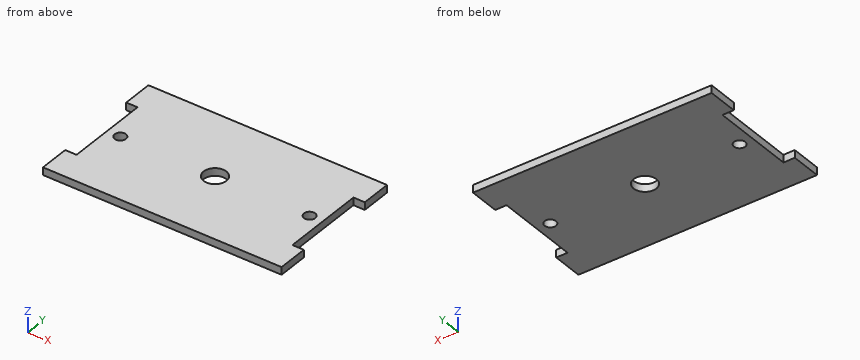
```python
from build123d import *

# Parameters (mm, degrees)
SKETCH_1_R      = 3
SKETCH_1_R_2    = 1.5
EXTRUDE_1_DEPTH = 2


with BuildPart() as part:
    # 草图1 → 凸台-拉伸1 (new body)
    with BuildSketch(Plane.XY):
        Polygon((-13.258857042, -42.872599913), (-16.258857042, -42.872599913), (-16.258857042, -50.872599913), (-13.258857042, -50.872599913), (-13.258857042, -72.872599913), (-16.258857042, -72.872599913), (-16.258857042, -80.872599913), (-13.258857042, -80.872599913), (43.741142958, -80.872599913), (46.741142958, -80.872599913), (46.741142958, -72.872599913), (43.741142958, -72.872599913), (43.741142958, -50.872599913), (46.741142958, -50.872599913), (46.741142958, -42.872599913), (43.741142958, -42.872599913), (15.241142958, -42.872599913), align=None)
        with Locations((15.241142958, -61.872599913)):
            Circle(SKETCH_1_R, mode=Mode.SUBTRACT)
        with Locations((40.241142958, -61.872599913)):
            Circle(SKETCH_1_R_2, mode=Mode.SUBTRACT)
        with Locations(Location((-9.758857042, -61.872599913, 0), (0, 0, 180))):
            Circle(SKETCH_1_R_2, mode=Mode.SUBTRACT)
    extrude(amount=EXTRUDE_1_DEPTH)


solid = part.part
```
Could you check a few things on this model? Use its own coordinates, in mm. Coordinates: 2 decimals unless noted, no trailing zeros. Loops run counter-clockwise (first coordinate to the right, second up) from the corner with the lowest first, then second, coordinate; pieces in that order, holes last.
1) Imagine slicing it at A-A (z = 0.55). List the corners of the cut face in (x, y) for me.
Reported:
outline: (-16.26, -80.87) - (46.74, -80.87) - (46.74, -72.87) - (43.74, -72.87) - (43.74, -50.87) - (46.74, -50.87) - (46.74, -42.87) - (-16.26, -42.87) - (-16.26, -50.87) - (-13.26, -50.87) - (-13.26, -72.87) - (-16.26, -72.87) - close; hole circle Ø3 at (-9.76, -61.87); hole circle Ø6 at (15.24, -61.87); hole circle Ø3 at (40.24, -61.87)
2) Imagine slicing it at B-B (y = -61). List the corners of the cut face in (x, z) for me, and give its area (3 significant figures).
Reported:
outline: (-13.26, 0) - (-10.98, 0) - (-10.98, 2) - (-13.26, 2) - close; (-8.54, 0) - (12.37, 0) - (12.37, 2) - (-8.54, 2) - close; (18.11, 0) - (39.02, 0) - (39.02, 2) - (18.11, 2) - close; (41.46, 0) - (43.74, 0) - (43.74, 2) - (41.46, 2) - close
area: 92.8 mm2
3) Imagine slicing it at D-D (y = -65.5). List the corners of the cut face in (x, z) for me.
Reported:
outline: (-13.26, 0) - (43.74, 0) - (43.74, 2) - (-13.26, 2) - close
4) Please list where these lines run through material, in increasing order: line 1 along X through (y, z) = (-61, 1.1); line 2 along X through (y, z) = (-53, 1.5); line 3 along Y through (x, z) = (14, 0.35).
Reported:
line 1: x = -13.26 to -10.98, -8.54 to 12.37, 18.11 to 39.02, 41.46 to 43.74
line 2: x = -13.26 to 43.74
line 3: y = -80.87 to -64.6, -59.14 to -42.87
5) Imagine slicing it at C-C (x = 40). List the corners of the cut face in (y, z) for me, and give its area (3 significant figures).
Reported:
outline: (-80.87, 0) - (-63.35, 0) - (-63.35, 2) - (-80.87, 2) - close; (-60.39, 0) - (-42.87, 0) - (-42.87, 2) - (-60.39, 2) - close
area: 70.1 mm2
6) Will these pins go through, and if not, where does the flat tip stop? pin 1 Ø1 at (y, z) = (-57.5, 1.5) entering from +X; pin 2 Ø2.5 at (x, y) = (40.24, -61.87) entering from +Z.
Reported:
pin 1: stops at x = 43.74
pin 2: passes through
